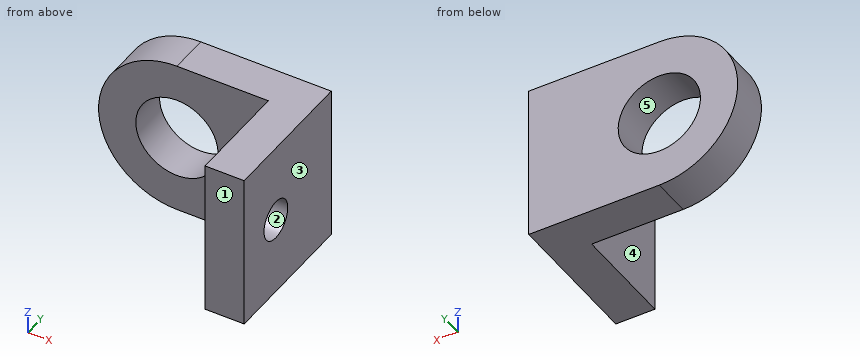
from build123d import *

# Parameters (mm, degrees)
SKETCH2_R           = 3.15
BOSS_EXTRUDE1_DEPTH = 3
SKETCH2_3_W         = 3
SKETCH2_3_H         = 6
BOSS_EXTRUDE2_DEPTH = 8
SKETCH4_R           = 1.5
CUT_EXTRUDE1_DEPTH  = 17.401219467


with BuildPart() as part:
    # Sketch2 → Boss-Extrude1 (new body)
    with BuildSketch(Plane(origin=(0, 0, 0), x_dir=(1, 0, 0), z_dir=(0, 1, 0))):
        with BuildLine():
            Line((0, 6), (10, 6))
            Line((10, 6), (10, -6))
            Line((10, -6), (0, -6))
            ThreePointArc((0, -6), (-6, 0), (0, 6))
        make_face()
        with Locations(Location((0, 0, 0), (0, 0, 270))):
            Circle(SKETCH2_R, mode=Mode.SUBTRACT)
    extrude(amount=BOSS_EXTRUDE1_DEPTH)

    # Sketch2_3 → Boss-Extrude2 (add)
    with BuildSketch(Plane(origin=(0, 0, 0), x_dir=(1, 0, 0), z_dir=(0, 1, 0))):
        with Locations((8.5, 3)):
            Rectangle(SKETCH2_3_W, SKETCH2_3_H)
        with Locations((8.5, -3)):
            Rectangle(SKETCH2_3_W, SKETCH2_3_H)
    extrude(amount=-BOSS_EXTRUDE2_DEPTH)

    # Sketch4 → Cut-Extrude1 (cut, through all)
    with BuildSketch(Plane.ZY.offset(-7)):
        with Locations((0, -4)):
            Circle(SKETCH4_R)
    extrude(amount=-CUT_EXTRUDE1_DEPTH, mode=Mode.SUBTRACT)


solid = part.part
Design review of the part built by this model. Coordinates are the model's own, in mm. Face numbers are marked on the shaded views. A direction names the side the tool comes from. Coordinates: 2 decimals unless noted, no trailing zeros. Write each loop counter-clockwise with the first axis right and the second up, starting at its lowest first coordinate (ties: lowest second). Pieces come first, ordered by that corner, then holes. Notation, with made-up numbers: (16.5, 56) - (52.5, 56) arc R12 cw to (52.5, 71) - close; hole circle Ø1 at (26.5, -1.5). An arc over 180 degrees is marked (long way). Use one line per item in the form item = value.
Q1. Machinability: for the marked faces 4 and 5, which of the approach directions +Z, -Z, +X, -X, +Y, -Y give a long, thin tool a straight path to every point of the face, cutting with its end or side? Answer none if there is none.
Taken from the geometry:
face_4 = +Z, -Z, -X, -Y
face_5 = +Y, -Y
Q2. Consider section D-D (z = -2.5). Write out the cut boundary in (x, y).
Taken from the geometry:
outline = (-5.45, 0) - (-1.92, 0) - (-1.92, 3) - (-5.45, 3) - close; (1.92, 0) - (7, 0) - (7, -8) - (10, -8) - (10, 3) - (1.92, 3) - close
Q3. Consider section B-B (z = 0). Write out the cut boundary in (x, y).
Taken from the geometry:
outline = (-6, 0) - (-3.15, 0) - (-3.15, 3) - (-6, 3) - close; (3.15, 0) - (7, 0) - (7, -2.5) - (10, -2.5) - (10, 3) - (3.15, 3) - close; (7, -8) - (10, -8) - (10, -5.5) - (7, -5.5) - close
Q4. The part is to be moulded in two halves that separate along Y. For the marked faces 1, 2 and 3, say which applies: +Y half, -Y half, draft (parallel to the pull), parting line (faces both ways), or undercut.
Taken from the geometry:
face_1 = -Y half
face_2 = undercut
face_3 = draft
Q5. Consider section A-A (y = -4). Write out the cut boundary in (x, z).
Taken from the geometry:
outline = (7, -6) - (10, -6) - (10, -1.5) - (7, -1.5) - close; (7, 1.5) - (10, 1.5) - (10, 6) - (7, 6) - close
Q6. Insertion check: pin 1 Ø5 at (x, z) = (0, 0) entering from -Y; pin 2 Ø4 at (y, z) = (-3.5, 2) entering from -X. Each pin has a flat end and moves straight along its axis. Give the tip position at first contact, or say it passes through.
Taken from the geometry:
pin_1 = through
pin_2 = 7
Q7. For probe 1 along X at (y, z) = (1.8, 0); probe 2 along X at (y, z) = (-0.5, 3); probe 3 along Y at (x, z) = (-4.25, 0.5), list the stretches that pass through material, from the lowest coordinate up.
Taken from the geometry:
probe_1 = -6 to -3.15, 3.15 to 10
probe_2 = 7 to 10
probe_3 = 0 to 3
Q8. Consider section C-C (x = -0.5). Write out the cut boundary in (y, z).
Taken from the geometry:
outline = (0, -5.98) - (3, -5.98) - (3, -3.11) - (0, -3.11) - close; (0, 3.11) - (3, 3.11) - (3, 5.98) - (0, 5.98) - close
